Build history of the part. All positions in model axes, mm. Round coordinates to 2 decimals unless told otherwise and drop trailing zeros. Use a Markdown table: item, result.
from build123d import *

# Parameters (mm, degrees)
SKETCH1_R           = 500
BOSS_EXTRUDE1_DEPTH = 20
BOSS_EXTRUDE1_TAPER = 45


with BuildPart() as part:
    # Sketch1 → Boss-Extrude1 (new body)
    with BuildSketch(Plane(origin=(0, 0, 0), x_dir=(1, 0, 0), z_dir=(0, 1, 0))):
        Circle(SKETCH1_R)
    extrude(amount=BOSS_EXTRUDE1_DEPTH, taper=BOSS_EXTRUDE1_TAPER)

    # Sweep1: sweep along a path in Sketch3
    with BuildLine(Plane(origin=(0, 0, 0), x_dir=(0, 0, -1), z_dir=(1, 0, 0))) as sweep1_path:
        ThreePointArc((480, 20), (238.376555203, 429.939732355), (-231.026329166, 508))
    # Sketch2 → Sweep1 (sweep)
    with BuildSketch(Plane(origin=(0, 20, 0), x_dir=(1, 0, 0), z_dir=(0, 1, 0))):
        with BuildLine():
            ThreePointArc((-462.894156368, 127), (0, 480), (462.894156368, 127))
            ThreePointArc((462.894156368, 127), (459.395258906, 120.855269204), (453.250528111, 124.354166667))
            ThreePointArc((453.250528111, 124.354166667), (0, 470), (-453.250528111, 124.354166667))
            ThreePointArc((-453.250528111, 124.354166667), (-459.395258906, 120.855269204), (-462.894156368, 127))
        make_face()
    sweep(path=sweep1_path.line)


solid = part.part
Q1. Drill centre lines: L1, parallel to Y at x = -39, z = 2; L2, parallel to Y at x = -57, z = 138; L3, parallel to Y at x = 1.5, z = 329. Where is each one in solid material? Low to high.
Response values:
| item | result |
|---|---|
| L1 | y = 0 to 20, 511.56 to 521.65 |
| L2 | y = 0 to 20, 512.18 to 522.27 |
| L3 | y = 0 to 20 |
Q2. Drop flat-ended pins along their axis: P1, Ø8, axis at x = -323, y = 413, coming from the +Z side; P2, Ø3, axis at y = 296.5, z = -89, coming from the +X side; P3, Ø1, axis at x = 203.5, z = -259.5, coming from the +Y side; P4, Ø1, axis at x = -17.5, y = 298.5, coming from the +Z side. Give the stop position or say it passes through.
Response values:
| item | result |
|---|---|
| P1 | passes through |
| P2 | stops at x = 385.74 |
| P3 | stops at y = 357.27 |
| P4 | stops at z = -360.72 |
Q3. Two-plate mould, pull along Y, no slides. Class faces 1 (the flat face through (-7, 0, -7)), 2 (the flat face through (-7, 20, -2)): +Y half, -Y half, draft (parallel to the pull), parting line (faces both ways), or undercut.
Response values:
| item | result |
|---|---|
| face 1 | -Y half |
| face 2 | undercut |
